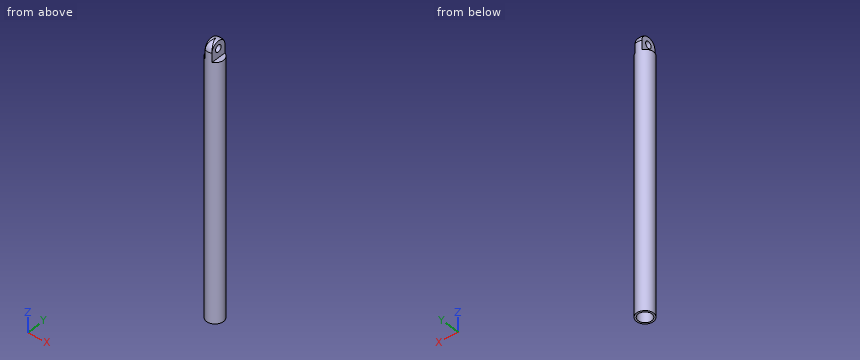
from build123d import *

# Parameters (mm, degrees)
SKETCH_1_R          = 75
EXTRUDE_1_DEPTH     = 2400
CUT_EXTRUDE_1_DEPTH = 150
SKETCH_3_R          = 30
CUT_EXTRUDE_2_DEPTH = 150
FILLET_1_R          = 70
SKETCH_4_R          = 60
CUT_EXTRUDE_4_DEPTH = 2200
SCALE_1_SCALE       = 0.345


with BuildPart() as part:
    # 草图1 → 凸台-拉伸1 (new body)
    with BuildSketch(Plane.XY):
        Circle(SKETCH_1_R)
    extrude(amount=EXTRUDE_1_DEPTH)

    # 草图2 → 切除-拉伸1 (cut)
    with BuildSketch(Plane.XY.offset(2400)):
        Polygon((-30, 75), (-30, -75), (-133.073279379, -42.369308492), (-77.396642949, 65.414797111), align=None)
        Polygon((30, 75), (30, -75), (106.458623503, -47.875789018), (106.458623503, 55.829594222), align=None)
    extrude(amount=-CUT_EXTRUDE_1_DEPTH, mode=Mode.SUBTRACT)

    # 草图3 → 切除-拉伸2 (cut)
    with BuildSketch(Plane(origin=(30, 0, 0), x_dir=(0, 0, -1), z_dir=(1, 0, 0))):
        with Locations((-2330, 0)):
            Circle(SKETCH_3_R)
    extrude(amount=-CUT_EXTRUDE_2_DEPTH, mode=Mode.SUBTRACT)

    # 圆角1
    # the kernel refuses this fillet: 70 mm, written as the material it takes off along each edge
    with BuildSketch(Plane(origin=(0, 0, 2400), x_dir=(0.3861785994276561, -0.922424029036589, 0), z_dir=(-0.922424029036589, -0.3861785994276561, 0))) as fillet_1_piece_1:
        with BuildLine():
            CenterArc((75 - FILLET_1_R, -FILLET_1_R), FILLET_1_R, 0, 90)
            Line((75 - FILLET_1_R, 0), (75, 0))
            Line((75, 0), (75, -FILLET_1_R))
        make_face()
    revolve(axis=Axis((0, 0, 2400), (0, 0, 1)), revolution_arc=314.566142673, mode=Mode.SUBTRACT)
    with BuildSketch(Plane(origin=(0, 0, 2400), x_dir=(-0.386178599427656, 0.922424029036589, 0), z_dir=(0.922424029036589, 0.386178599427656, 0))) as fillet_1_piece_2:
        with BuildLine():
            CenterArc((75 - FILLET_1_R, -FILLET_1_R), FILLET_1_R, 0, 90)
            Line((75 - FILLET_1_R, 0), (75, 0))
            Line((75, 0), (75, -FILLET_1_R))
        make_face()
    revolve(axis=Axis((0, 0, 2400), (0, 0, 1)), revolution_arc=314.566142673, mode=Mode.SUBTRACT)

    # 草图4 → 切除-拉伸4 (cut)
    with BuildSketch(Plane(origin=(0, 0, 0), x_dir=(-1, 0, 0), z_dir=(0, 0, -1))):
        Circle(SKETCH_4_R)
    extrude(amount=-CUT_EXTRUDE_4_DEPTH, mode=Mode.SUBTRACT)


with BuildPart() as part_1:
    # 缩放比例1: scaled about (0, 0, 0)
    add(part.part.scale(SCALE_1_SCALE))


solid = part_1.part
Build history of the part. All positions in model axes, mm. Coordinates: 2 decimals unless noted, no trailing zeros. Write each loop counter-clockwise with the first axis right and the second up, starting at its lowest first coordinate (ties: lowest second). Pieces come first, ordered by that corner, then holes. Notation, with made-up numbers: (-4, 40) -> (34, 40) arc R25 cw to (34, 74) -> close; hole circle Ø3 at (-35, 19.5). An arc over 180 degrees is marked (long way). Use CSV: the item, a comma, the result in double quotes. Start each with the question number.
Q1. Cut at A-A, the plane z = 339. List the corners of the cut face in (x, y) (3 decimals), then the cut area to 3 significant figures.
Q2. Drill centre lines: probe 1 along Y at (x, z) = (0, 174.5) (3 decimals); probe 2 along Z at (x, y) = (18.5, 16); probe 3 along Z at (x, y) = (10.5, 14). Where is each one in solid material? Low to high.
Q3. Flat gauge pins, fed straight in: pin 1 Ø12 at (x, y) = (15, -3) entering from +Z; pin 2 Ø1.5 at (y, z) = (-8, 719.5) entering from -X; pin 3 Ø1 at (x, y) = (-9.5, -3.5) entering from +Z. Where does each tip first touch, or does it go through?
Checked values:
1,outline,"circle Ø51.75 at (0, 0); hole circle Ø41.4 at (0, 0)"
1,area,"757 mm²"
2,probe 1,"y = -25.875 to -20.7, 20.7 to 25.875"
2,probe 2,"z = 0 to 776.25"
2,probe 3,"z = 759 to 776.25"
3,pin 1,"stops at z = 826.78"
3,pin 2,"stops at x = -24.84"
3,pin 3,"stops at z = 826.67"
